The model under review builds one solid part; all positions refer to its coordinate system, in mm. A direction names the side the tool comes from. Coordinates: 2 decimals unless noted, no trailing zeros. Loops run counter-clockwise (first coordinate to the right, second up) from the corner with the lowest first, then second, coordinate; pieces in that order, holes last. Notation, with made-up numbers: M -4.75,-2 L 14.25,-2 A23 cw 14.25,32 Z; hole C 21.25,65.5 d3. An arc over 180 degrees is marked long. Write item = value, one per line. Start each with the question number.
Q1. Mouldability with a two-part tool opening along X and no side actions: class faces 1 (the face through (12, 2, 4)), 2 (the face through (-3, 1, 7.8)), 3 (the face through (13, 3, 7.8)), 4 (the face through (11.25, 4, 4)) as released by +X, released by -X, zero draft, split by the parting line, or undercut.
Q2. We need section D-D on x = -2. Give the boundary of the cut face in (y, z), and give its area (3 significant figures).
Q3. We need section B-B on z = 7.5. Give the boundary of the cut face in (x, y), and give its area (3 significant figures).
Q4. Clearance check with flat-ended pins moving along their axes: pin 1 Ø2 at (x, y) = (-14, 3) entering from -Z; pin 2 Ø1 at (y, z) = (1, 4) entering from +X; pin 3 Ø1.6 at (x, y) = (-19.5, 3.5) entering from -Z; pin 4 Ø1.4 at (y, z) = (2.5, 5.5) entering from -X. State where each tip first meets the part, or that it passes through.
Q5. We need section C-C on y = 0.95. Give the boundary of the cut face in (x, z), and give its area (3 significant figures).
Q6. For faces 5 (the face through (-18, 4.67, 5)), 6 (the face through (-19, 2, 7.8)), 7 (the face through (-3, 2.3, 4)), 8 (the face through (-19, 2, 8.8)), list the 3-axis set-ups (+Z, -Z, +X, -X, +Y, -Y) from which the entire face can be reached by the end or side of a thin tool; tool diameter is ignored.
Q7. Wall thickness on probe 1 along X at (y, z) = (3.2, 2); probe 2 along Z at (x, y) = (-12, 2.2); probe 3 along Y at (x, z) = (-12, 5.5): over which ranges is each line inside the solid? List them lowest first.
Q8. We need section A-A on y = 3.25. Give the boundary of the cut face in (x, z), and give its area (3 significant figures).
from build123d import *

# Parameters (mm, degrees)
F1_DEPTH = 7.8
F3_DEPTH = 1
F4_W     = 28.8
F4_H     = 1
F5_DEPTH = 5.001


with BuildPart() as f1:
    # F0 (on Top) → F1 (new body)
    with BuildSketch(Plane.XY):
        Polygon((-18.3, 4.669697), (-18.3, 0), (12, 0), (12, 5), (11.25, 5), (11.25, 2.3), (-17.55, 2.3), (-17.55, 4.669697), align=None)
    extrude(amount=F1_DEPTH)

    # F2 (on face) → F3 (join)
    with BuildSketch(Plane.XY.offset(7.8)):
        Polygon((-17.55, 2.3), (-17.55, 4.669697), (-19.8, 4.669697), (-19.8, 0), (13.5, 0), (13.5, 5), (11.25, 5), (11.25, 2.3), align=None)
    extrude(amount=F3_DEPTH)

    # F4 (on face) → F5 (cut, through all)
    with BuildSketch(Plane.XZ):
        with Locations((-3.15, 8.3)):
            Rectangle(F4_W, F4_H)
    extrude(amount=-F5_DEPTH, mode=Mode.SUBTRACT)


solid = f1.part
Returned:
q1.face_1 = released by +X
q1.face_2 = undercut
q1.face_3 = zero draft
q1.face_4 = undercut
q2.outline = M 0,0 L 2.3,0 L 2.3,7.8 L 0,7.8 Z
q2.area = 17.9 mm^2
q3.outline = M -18.3,0 L 12,0 L 12,5 L 11.25,5 L 11.25,2.3 L -17.55,2.3 L -17.55,4.67 L -18.3,4.67 Z
q3.area = 73.5 mm^2
q4.pin_1 = 0
q4.pin_2 = 12
q4.pin_3 = 7.8
q4.pin_4 = -18.3
q5.outline = M -19.8,7.8 L -18.3,7.8 L -18.3,0 L 12,0 L 12,7.8 L 13.5,7.8 L 13.5,8.8 L 11.25,8.8 L 11.25,7.8 L -17.55,7.8 L -17.55,8.8 L -19.8,8.8 Z
q5.area = 241 mm^2
q6.face_5 = +Z, -Z, -X, +Y
q6.face_6 = -Z, -X, +Y, -Y
q6.face_7 = +Z, -Z, +Y
q6.face_8 = +Z, +X, -X, +Y, -Y
q7.probe_1 = -18.3 to -17.55, 11.25 to 12
q7.probe_2 = 0 to 7.8
q7.probe_3 = 0 to 2.3
q8.outline = M -19.8,7.8 L -18.3,7.8 L -18.3,0 L -17.55,0 L -17.55,8.8 L -19.8,8.8 Z; M 11.25,0 L 12,0 L 12,7.8 L 13.5,7.8 L 13.5,8.8 L 11.25,8.8 Z
q8.area = 16.2 mm^2
